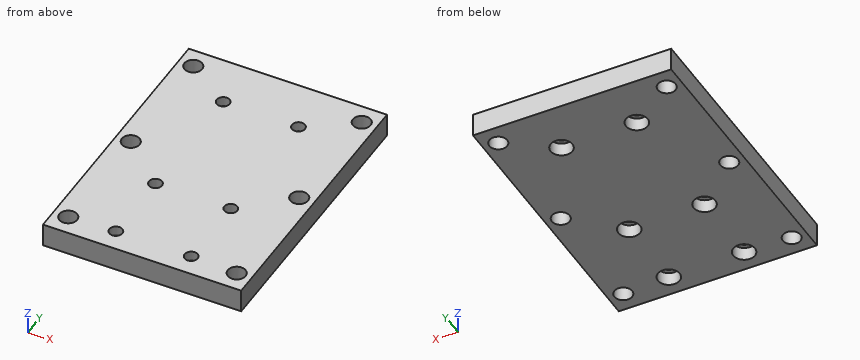
from build123d import *

# Parameters (mm, degrees)
SKETCH_1_W                  = 100
SKETCH_1_H                  = 140
SKETCH_1_R                  = 4.5
EXTRUDE_1_DEPTH             = 12
HOLE_WIZARD_1_D             = 6.6
HOLE_WIZARD_1_CBORE_D       = 11
HOLE_WIZARD_1_CBORE_DEPTH   = 6.8
PATTERN_LINEAR_1_COUNT      = 2
PATTERN_LINEAR_1_PITCH      = 38
PATTERN_LINEAR_1_COUNT_DIR2 = 2
PATTERN_LINEAR_1_PITCH_DIR2 = 38
HOLE_WIZARD_0_D             = 6.6
HOLE_WIZARD_0_CBORE_D       = 11
HOLE_WIZARD_0_CBORE_DEPTH   = 6.8
PATTERN_LINEAR_2_COUNT      = 2
PATTERN_LINEAR_2_PITCH      = 38


with BuildPart() as part:
    # 草图1 → 凸台-拉伸1 (new body)
    with BuildSketch(Plane.XY):
        Rectangle(SKETCH_1_W, SKETCH_1_H)
        with Locations((-42.5, -60)):
            Circle(SKETCH_1_R, mode=Mode.SUBTRACT)
        with Locations((42.5, -60)):
            Circle(SKETCH_1_R, mode=Mode.SUBTRACT)
        with Locations((42.5, 0)):
            Circle(SKETCH_1_R, mode=Mode.SUBTRACT)
        with Locations((42.5, 60)):
            Circle(SKETCH_1_R, mode=Mode.SUBTRACT)
        with Locations((-42.5, 0)):
            Circle(SKETCH_1_R, mode=Mode.SUBTRACT)
        with Locations((-42.5, 60)):
            Circle(SKETCH_1_R, mode=Mode.SUBTRACT)
    extrude(amount=EXTRUDE_1_DEPTH)

    # 打孔尺寸(%根据)内六角圆柱头螺钉的类型1 (through all)
    with Locations(Plane(origin=(0, 0, 0), x_dir=(-1, 0, 0), z_dir=(0, 0, -1))):
        with Locations((-19, -59)):
            hole_wizard_1 = CounterBoreHole(HOLE_WIZARD_1_D / 2, HOLE_WIZARD_1_CBORE_D / 2, HOLE_WIZARD_1_CBORE_DEPTH)

    # 阵列(线性)1: Hole Wizard 1 2 × 2
    with Locations(*[(-j * PATTERN_LINEAR_1_PITCH_DIR2, i * PATTERN_LINEAR_1_PITCH, 0) for i in range(PATTERN_LINEAR_1_COUNT) for j in range(PATTERN_LINEAR_1_COUNT_DIR2) if (i, j) != (0, 0)]):
        add(hole_wizard_1, mode=Mode.SUBTRACT)

    # 打孔尺寸(%根据)内六角圆柱头螺钉的类型0 (through all)
    with Locations(Plane(origin=(0, 0, 0), x_dir=(-1, 0, 0), z_dir=(0, 0, -1))):
        with Locations((-19, 44)):
            hole_wizard_0 = CounterBoreHole(HOLE_WIZARD_0_D / 2, HOLE_WIZARD_0_CBORE_D / 2, HOLE_WIZARD_0_CBORE_DEPTH)

    # 阵列(线性)2: 打孔尺寸(%根据)内六角圆柱头螺钉的类型0 ×2
    with Locations(*[(-i * PATTERN_LINEAR_2_PITCH, 0, 0) for i in range(1, PATTERN_LINEAR_2_COUNT)]):
        add(hole_wizard_0, mode=Mode.SUBTRACT)


solid = part.part
Design review of the part built by this model. Coordinates are the model's own, in mm. Give positions to 0.01 mm unless a question says otherwise; leave off trailing zeros. Write each loop counter-clockwise with the first axis right and the second up, starting at its lowest first coordinate (ties: lowest second). Pieces come first, ordered by that corner, then holes. Notation, with made-up numbers: M 62.25,5 L 97.25,5 A6 cw 97.25,9 Z; hole C 81.25,-25.75 d11. An arc over 180 degrees is marked long. Return JSON: item names as keys, results as strings. Group by question number.
Item 1: Take a section at A-A (x = -19). Give the boundary of the cut face in (y, z).
Item 2: Take a section at B-B (z = 8.5). Count the separate pieces of the cut face and the enclosed holes in it, plus the area to 3 significant figures.
Item 3: Take a section at C-C (y = 60). Give the boundary of the cut face in (x, z), plus the area to 3 significant figures.
Item 4: Clearance check with flat-ended pins moving along their axes: pin 1 Ø17.5 at (x, y) = (19, 44) entering from +Z; pin 2 Ø3.5 at (x, y) = (-20.5, 46.5) entering from -Z. State where each tip first meets the part, or that it passes through.
Item 5: Take a section at D-D (x = 42.5). Give the boundary of the cut face in (y, z), plus the area to 3 significant figures.
Item 6: Wall thickness on line 1 along Y through (x, z) = (42.5, 7.5); line 2 along X through (y, z) = (-17.5, 4.25); line 3 along X through (y, z) = (-61, 4): over which ranges is each line inside the solid? List them lowest first.
Return value:
{
 "1": {"outline": "M -70,0 L -64.5,0 L -64.5,6.8 L -62.3,6.8 L -62.3,12 L -70,12 Z; M -55.7,6.8 L -53.5,6.8 L -53.5,0 L -26.5,0 L -26.5,6.8 L -24.3,6.8 L -24.3,12 L -55.7,12 Z; M -17.7,6.8 L -15.5,6.8 L -15.5,0 L 38.5,0 L 38.5,6.8 L 40.7,6.8 L 40.7,12 L -17.7,12 Z; M 47.3,6.8 L 49.5,6.8 L 49.5,0 L 70,0 L 70,12 L 47.3,12 Z"},
 "2": {"separate pieces": "1", "enclosed holes": "12", "area": "13,400 mm2"},
 "3": {"outline": "M -50,0 L -47,0 L -47,12 L -50,12 Z; M -38,0 L 38,0 L 38,12 L -38,12 Z; M 47,0 L 50,0 L 50,12 L 47,12 Z", "area": "984 mm2"},
 "4": {"pin 1": "stops at z = 12", "pin 2": "stops at z = 6.8"},
 "5": {"outline": "M -70,0 L -64.5,0 L -64.5,12 L -70,12 Z; M -55.5,0 L -4.5,0 L -4.5,12 L -55.5,12 Z; M 4.5,0 L 55.5,0 L 55.5,12 L 4.5,12 Z; M 64.5,0 L 70,0 L 70,12 L 64.5,12 Z", "area": "1,360 mm2"},
 "6": {"line 1": "y = -70 to -64.5, -55.5 to -4.5, 4.5 to 55.5, 64.5 to 70", "line 2": "x = -50 to -23.24, -14.76 to 14.76, 23.24 to 50", "line 3": "x = -50 to -46.89, -38.11 to -24.12, -13.88 to 13.88, 24.12 to 38.11, 46.89 to 50"}
}
